Verification items for the finished model (mm, model axes). Round coordinates to 2 decimals unless told otherwise and drop trailing zeros. Loops run counter-clockwise (first coordinate to the right, second up) from the corner with the lowest first, then second, coordinate; pieces in that order, holes last.
Autodesk Inventor part; units mm, degrees
ref_plane "YZ Plane" through (0, 0, 0) normal (1, 0, 0) x (0, 1, 0)
ref_plane "XZ Plane" through (0, 0, 0) normal (0, 1, 0) x (-1, 0, 0)
ref_plane "XY Plane" through (0, 0, 0) normal (0, 0, 1) x (1, 0, 0)
sketch "Sketch1" plane through (0, 0, 0) normal (1, 0, 0) x (0, 1, 0)
  line L0 (-4.0415, 0) -> (-2.0207, 3.5)
  line L1 (-2.0207, 3.5) -> (2.0207, 3.5)
  line L2 (2.0207, 3.5) -> (4.0415, 0)
  line L3 (4.0415, 0) -> (2.0207, -3.5)
  line L4 (2.0207, -3.5) -> (-2.0207, -3.5)
  line L5 (-2.0207, -3.5) -> (-4.0415, 0)
  point P0 (0, 0)
  point P1 (0, 0)
  dimension "d0" = 8.0829
extrude "Body" add sketch "Sketch1" along normal blind 3.1
sketch "Sketch2" plane through (0, 0, 0) normal (0, 0, 1) x (1, 0, 0)
  line L0 (0, 2.0207) -> (0, 4.0415)
  line L1 (0, 4.0415) -> (3.1, 4.0415)
  line L2 (3.1, 2.0207) -> (3.1, 4.0415)
  line L3 (-0.62, 0) -> (3.72, 0)
  line L4 (0.3126, 4.0415) -> (0, 3.5)
  line L5 (2.7874, 4.0415) -> (3.1, 3.5)
  dimension "d3" = 30
  dimension "d4" = 30
  dimension "d5" = 7
  dimension "d6" = 7
revolve "Chamfer1" cut sketch "Sketch2" angle 360 about axis through (-10, 0, 0) along (1, 0, 0)
sketch "Sketch3" plane through (3.1, 0, 0) normal (1, 0, 0) x (0, 0, -1)
  arc A0 (-1.75, -3.0311) -> (1.75, -3.0311) centre (0, 0) ccw
hole "Thread" at (3.1, 0, 0) direction (-1, 0, 0) diameter 3.242 end through all
chamfer "Chamfer2" distance 0.3789 angle 30 1 edges at (3.1, 0, 1.621) measured on face at (3.1, 2.8569, -0.0651)
chamfer "Chamfer3" distance 0.3789 angle 30 1 edges at (0, 0, 1.621) measured on face at (0, 2.8569, -0.0651)
equation "\"d0\" = 1.1547 * SW"
equation "\"d8\" = -0.5 * GD1 + 0.5 * NND"
equation "\"d40\" = -0.5 * GD1 + 0.5 * NND"
equation "\"d10\" = -0.5 * GD1 + 0.5 * NND"
equation "\"d41\" = -0.5 * GD1 + 0.5 * NND"
equation "\"d3\" = ANG1"
equation "\"d4\" = ANG2"
equation "\"d5\" = SW0"
equation "\"d6\" = SW01"
equation "\"ANG1\" = 30deg"
equation "\"ANG2\" = 30deg"
equation "\"NND\" = 4"
equation "\"KOH\" = 3.8"
equation "\"SW\" = 7"
equation "\"SW0\" = SW"
equation "\"SW01\" = SW"
equation "\"E0\" = 1.155 * SW"
equation "\"THREADDIA\" = 4"
equation "\"TPU\" = 0.7"
equation "\"GUL\" = 0.541266 * TPU"
equation "\"GAL\" = 0.541266 * TPU"
equation "\"PTC\" = TPU"
equation "\"TOA\" = 30deg"
properties part number "NUT, HEX, M4" material "Steel, MS"
1. Gauge pin test, flat ends, axial feed: P1, Ø1.9, axis at y = 0, z = 0, coming from the -X side; P2, Ø2, axis at y = 0.5, z = 2, coming from the -X side. Record the tip position at first contact, or that the pin passes through.
2. Section check A-A (x = 2.5). Enter the section's corners in (y, z), then the cut area to 3 significant figures.
3. Release check for a two-part mould opening along Z. For faces 1 (the face through (1.531, 1.438, -0.748)), 2 (the face through (3.024, 1.808, 3.15)), 3 (the face through (2, 0, -3.5)), 4 (the face through (3.024, -3.632, -0.009)) record: released by +Z, released by -Z, zero draft, split by the parting line, or undercut.
4. Scan lines: L1, parallel to Z at x = 1.05, y = 0; L2, parallel to Z at x = 2.3, y = 1.25; L3, parallel to Y at x = 1.8, z = 0.75. Record each from-to range of solid material in increasing order.
Taken from the geometry:
1. P1: passes through
1. P2: stops at x = 0
2. outline: (-4.04, 0) - (-2.02, -3.5) - (2.02, -3.5) - (4.04, 0) - (2.02, 3.5) - (-2.02, 3.5) - close; hole circle Ø3.24 at (0, 0)
2. area: 34.2 mm2
3. face 1: undercut
3. face 2: released by +Z
3. face 3: released by -Z
3. face 4: split by the parting line
4. L1: z = -3.5 to -1.62, 1.62 to 3.5
4. L2: z = -3.5 to -1.03, 1.03 to 3.5
4. L3: y = -3.61 to -1.44, 1.44 to 3.61
